```python
from build123d import *

# Parameters (mm, degrees)
SKETCH1_W           = 355.6
SKETCH1_H           = 50.8
BOSS_EXTRUDE1_DEPTH = 4.7625
SKETCH2_W           = 6.858
SKETCH2_H           = 19.471321321
SKETCH2_W_2         = 6.35
SKETCH2_H_2         = 18.963321321
CUT_EXTRUDE1_DEPTH  = 180.668253752
SKETCH3_W           = 1.5875
SKETCH3_H           = 15.707678679
SKETCH3_H_2         = 15.621
CUT_EXTRUDE2_DEPTH  = 180.668253752
SKETCH4_W           = 0.3175
SKETCH4_H           = 19.471321321
BOSS_EXTRUDE2_DEPTH = 4.7625
SKETCH5_W           = 0.3175
SKETCH5_H           = 19.471321321
CUT_EXTRUDE4_DEPTH  = 179.097407512


with BuildPart() as part:
    # Sketch1 → Boss-Extrude1 (new body)
    with BuildSketch(Plane(origin=(0, 0, 0), x_dir=(1, 0, 0), z_dir=(0, 1, 0))):
        Rectangle(SKETCH1_W, SKETCH1_H)
    extrude(amount=BOSS_EXTRUDE1_DEPTH)

    # Sketch2 → Cut-Extrude1 (cut, through all)
    with BuildSketch(Plane(origin=(0, 0, 0), x_dir=(-1, 0, 0), z_dir=(0, -1, 0))):
        with Locations((174.625, 0.043339339)):
            Rectangle(SKETCH2_W, SKETCH2_H)
        with Locations((174.625, 0.04333934)):
            Rectangle(SKETCH2_W_2, SKETCH2_H_2, mode=Mode.SUBTRACT)
        with Locations((79.375, 0.043339339)):
            Rectangle(SKETCH2_W, SKETCH2_H)
        with Locations((79.375, 0.04333934)):
            Rectangle(SKETCH2_W_2, SKETCH2_H_2, mode=Mode.SUBTRACT)
        with Locations((-79.375, 0.043339339)):
            Rectangle(SKETCH2_W, SKETCH2_H)
        with Locations((-79.375, 0.04333934)):
            Rectangle(SKETCH2_W_2, SKETCH2_H_2, mode=Mode.SUBTRACT)
        with Locations((-174.625, 0.043339339)):
            Rectangle(SKETCH2_W, SKETCH2_H)
        with Locations((-174.625, 0.04333934)):
            Rectangle(SKETCH2_W_2, SKETCH2_H_2, mode=Mode.SUBTRACT)
    extrude(amount=-CUT_EXTRUDE1_DEPTH, mode=Mode.SUBTRACT)


with BuildPart() as body_2:
    # of the pieces the cut leaves, the one that is kept (cut_extrude1_keep)
    add(part.part.solids().sort_by_distance((-177.8, 0, -25.4))[0])

    # Sketch3 → Cut-Extrude2 (cut, through all)
    with BuildSketch(Plane(origin=(0, 4.7625, 0), x_dir=(1, 0, 0), z_dir=(0, 1, 0))):
        with Locations((-177.00625, -17.546160661)):
            Rectangle(SKETCH3_W, SKETCH3_H)
        with Locations((-177.00625, 17.5895)):
            Rectangle(SKETCH3_W, SKETCH3_H_2)
        with Locations((177.00625, -17.546160661)):
            Rectangle(SKETCH3_W, SKETCH3_H)
        with Locations((177.00625, 17.5895)):
            Rectangle(SKETCH3_W, SKETCH3_H_2)
    extrude(amount=-CUT_EXTRUDE2_DEPTH, mode=Mode.SUBTRACT)

    # Sketch4 → Boss-Extrude2 (add)
    with BuildSketch(Plane(origin=(0, 4.7625, 0), x_dir=(1, 0, 0), z_dir=(0, 1, 0))):
        with Locations((-76.10475, 0.043339339)):
            Rectangle(SKETCH4_W, SKETCH4_H)
        with Locations((76.10475, 0.043339339)):
            Rectangle(SKETCH4_W, SKETCH4_H)
    extrude(amount=-BOSS_EXTRUDE2_DEPTH)

    # Sketch5 → Cut-Extrude4 (cut, through all)
    with BuildSketch(Plane(origin=(0, 4.7625, 0), x_dir=(1, 0, 0), z_dir=(0, 1, 0))):
        with Locations((-82.96275, 0.043339339)):
            Rectangle(SKETCH5_W, SKETCH5_H)
        with Locations((82.96275, 0.043339339)):
            Rectangle(SKETCH5_W, SKETCH5_H)
    extrude(amount=-CUT_EXTRUDE4_DEPTH, mode=Mode.SUBTRACT)


solid = body_2.part
```
The listing builds one solid part. Answer for the finished solid, in the listing's coordinates (mm). Round coordinates to 2 decimals unless told otherwise and drop trailing zeros. Loops run counter-clockwise (first coordinate to the right, second up) from the corner with the lowest first, then second, coordinate; pieces in that order, holes last.
Q1. Given pin 1 Ø1.4 at (y, z) = (3, 3) entering from -X; pin 2 Ø1.5 at (y, z) = (2, 0.5) entering from +X, each flat-ended and moving along its own axis, determine where each tip first touches the part or whether it passes through.
Q2. Find the intervals of material crossed by line 1 (X direction, y = 2.7, z = 6); line 2 (Z direction, x = 78.5, y = 0.95), in increasing order.
Q3. Section B-B, the plane z = -3.5 is taken. Determine the outline of the cut face in (x, y), then the cut area to 3 significant figures.
Q4. Section A-A, the plane y = 2.1 is taken. Determine the outline of the cut face in (x, z), then the cut area to 3 significant figures.
Completed:
1. pin 1: stops at x = -171.2
1. pin 2: stops at x = 171.2
2. line 1: x = -171.2 to -83.12, -76.26 to 76.26, 83.12 to 171.2
2. line 2: z = -25.4 to -9.78, 9.69 to 25.4
3. outline: (-171.2, 0) - (-83.12, 0) - (-83.12, 4.76) - (-171.2, 4.76) - close; (-76.26, 0) - (76.26, 0) - (76.26, 4.76) - (-76.26, 4.76) - close; (83.12, 0) - (171.2, 0) - (171.2, 4.76) - (83.12, 4.76) - close
3. area: 1,570 mm2
4. outline: (-176.21, -25.4) - (176.21, -25.4) - (176.21, -9.78) - (171.2, -9.78) - (171.2, 9.69) - (176.21, 9.69) - (176.21, 25.4) - (-176.21, 25.4) - (-176.21, 9.69) - (-171.2, 9.69) - (-171.2, -9.78) - (-176.21, -9.78) - close; hole (-83.12, -9.78) - (-76.26, -9.78) - (-76.26, 9.69) - (-83.12, 9.69) - close; hole (76.26, -9.78) - (83.12, -9.78) - (83.12, 9.69) - (76.26, 9.69) - close
4. area: 17,400 mm2
